from build123d import *

# Parameters (mm, degrees)
SKETCH1_W           = 30.746
SKETCH1_H           = 10.746
SKETCH1_W_2         = 29.246
SKETCH1_H_2         = 9.246
BOSS_EXTRUDE1_DEPTH = 8
SKETCH2_W           = 32.246
SKETCH2_H           = 12.246
BOSS_EXTRUDE2_DEPTH = 1
FILLET2_R           = 0.25
FILLET3_R           = 2
FILLET4_R           = 1
FILLET5_R           = 0.25


with BuildPart() as part:
    # Sketch1 → Boss-Extrude1 (new body)
    with BuildSketch(Plane.XY):
        with Locations((0, 38)):
            Rectangle(SKETCH1_W, SKETCH1_H)
        with Locations((0, 38)):
            Rectangle(SKETCH1_W_2, SKETCH1_H_2, mode=Mode.SUBTRACT)
    extrude(amount=BOSS_EXTRUDE1_DEPTH)

    # Sketch2 → Boss-Extrude2 (add)
    with BuildSketch(Plane.XY.offset(8)):
        with Locations((0, 38)):
            Rectangle(SKETCH2_W, SKETCH2_H)
    extrude(amount=BOSS_EXTRUDE2_DEPTH)

    # Fillet2
    fillet2_edges = [part.edges().sort_by_distance(p)[0] for p in [
        (-15.373, 43.373, 4),
        (15.373, 43.373, 4),
        (15.373, 32.627, 4),
        (-15.373, 32.627, 4),
    ]]
    fillet(fillet2_edges, radius=FILLET2_R)

    # Fillet3
    fillet3_edges = [part.edges().sort_by_distance(p)[0] for p in [
        (-16.123, 31.877, 8.5),
        (16.123, 31.877, 8.5),
        (16.123, 44.123, 8.5),
        (-16.123, 44.123, 8.5),
    ]]
    fillet(fillet3_edges, radius=FILLET3_R)

    # Fillet4
    fillet4_edges = [part.edges().sort_by_distance(p)[0] for p in [
        (14.623, 33.377, 4),
        (14.623, 42.623, 4),
        (-14.623, 42.623, 4),
        (-14.623, 33.377, 4),
    ]]
    fillet(fillet4_edges, radius=FILLET4_R)

    # Fillet5
    fillet5_edges = [part.edges().sort_by_distance(p)[0] for p in [
        (0, 44.123, 9),
        (16.123, 38, 9),
        (0, 31.877, 9),
        (-16.123, 38, 9),
        (-15.537213562, 43.537213562, 9),
        (-15.537213562, 32.462786438, 9),
        (15.537213562, 32.462786438, 9),
        (15.537213562, 43.537213562, 9),
    ]]
    fillet(fillet5_edges, radius=FILLET5_R)


solid = part.part
The model under review builds one solid part; all positions refer to its coordinate system, in mm. A direction names the side the tool comes from. Round coordinates to 2 decimals unless told otherwise and drop trailing zeros. Loops run counter-clockwise (first coordinate to the right, second up) from the corner with the lowest first, then second, coordinate; pieces in that order, holes last. Notation, with made-up numbers: (62, 23.25) -> (86, 23.25) arc R17 cw to (86, 32.25) -> close; hole circle Ø10 at (-29, 47). An arc over 180 degrees is marked (long way). Write item = value, one per line. Start each with the question number.
Item 1: Take a section at C-C on x = -2.5. Give the boundary of the cut face in (y, z).
Item 2: Insertion check: pin 1 (4 mm diameter, centred on x = 1.5, z = 4.5, fed in from +Y); pin 2 (2 mm diameter, centred on x = 0.5, z = 5, fed in from -Y); pin 3 (2.5 mm diameter, centred on y = 39, z = 4, fed in from -X). Each pin has a flat end and moves straight along its axis. Give the tip position at first contact, or say it passes through.
Item 3: To check wall thickness, follow L1, parallel to X at y = 40.5, z = 5.25; L2, parallel to Y at x = -8, z = 6.5; L3, parallel to X at y = 33.25, z = 7.5. State the ranges of each line that lie inside material, in increasing order.
Item 4: Mouldability with a two-part tool opening along Y and no side actions: class faces 5 (the flat face through (15.373, 38, 4)), 6 (the flat face through (14.623, 38, 4)), 7 (the cylindrical face through (-15.553, 32.478, 8.38)), 8 (the flat face through (0, 42.623, 4)) as released by +Y, released by -Y, zero draft, split by the parting line, or undercut.
Item 5: For faces 1 (the flat face through (0, 43.373, 4)), 2 (the flat face through (-15.373, 38, 4)), 3 (the flat face through (0, 32.627, 4)), 4 (the cylindrical face through (-14.32, 42.34, 4.06)), list the 3-axis set-ups (+Z, -Z, +X, -X, +Y, -Y) from which the entire face can be reached by the end or side of a thin tool; tool diameter is ignored.
Item 6: Take a section at B-B on y = 37.25. Give the boundary of the cut face in (x, z).
Item 7: Take a section at A-A on z = 3. Give the boundary of the cut face in (x, y).
Result:
q1.outline = (31.88, 8) -> (32.63, 8) -> (32.63, 0) -> (33.38, 0) -> (33.38, 8) -> (42.62, 8) -> (42.62, 0) -> (43.37, 0) -> (43.37, 8) -> (44.12, 8) -> (44.12, 8.75) arc R0.25 ccw to (43.87, 9) -> (32.13, 9) arc R0.25 ccw to (31.88, 8.75) -> close
q2.pin_1 = 43.37
q2.pin_2 = 32.63
q2.pin_3 = -15.37
q3.L1 = -15.37 to -14.62, 14.62 to 15.37
q3.L2 = 32.63 to 33.38, 42.62 to 43.37
q3.L3 = -15.37 to 15.37
q4.face_5 = zero draft
q4.face_6 = undercut
q4.face_7 = released by -Y
q4.face_8 = undercut
q5.face_1 = -Z, +X, -X, +Y
q5.face_2 = -Z, -X, +Y, -Y
q5.face_3 = -Z, +X, -X, -Y
q5.face_4 = -Z
q6.outline = (-16.12, 8) -> (-15.37, 8) -> (-15.37, 0) -> (-14.62, 0) -> (-14.62, 8) -> (14.62, 8) -> (14.62, 0) -> (15.37, 0) -> (15.37, 8) -> (16.12, 8) -> (16.12, 8.75) arc R0.25 ccw to (15.87, 9) -> (-15.87, 9) arc R0.25 ccw to (-16.12, 8.75) -> close
q7.outline = (-15.37, 32.88) arc R0.25 ccw to (-15.12, 32.63) -> (15.12, 32.63) arc R0.25 ccw to (15.37, 32.88) -> (15.37, 43.12) arc R0.25 ccw to (15.12, 43.37) -> (-15.12, 43.37) arc R0.25 ccw to (-15.37, 43.12) -> close; hole (-14.62, 34.38) arc R1 ccw to (-13.62, 33.38) -> (13.62, 33.38) arc R1 ccw to (14.62, 34.38) -> (14.62, 41.62) arc R1 ccw to (13.62, 42.62) -> (-13.62, 42.62) arc R1 ccw to (-14.62, 41.62) -> close
